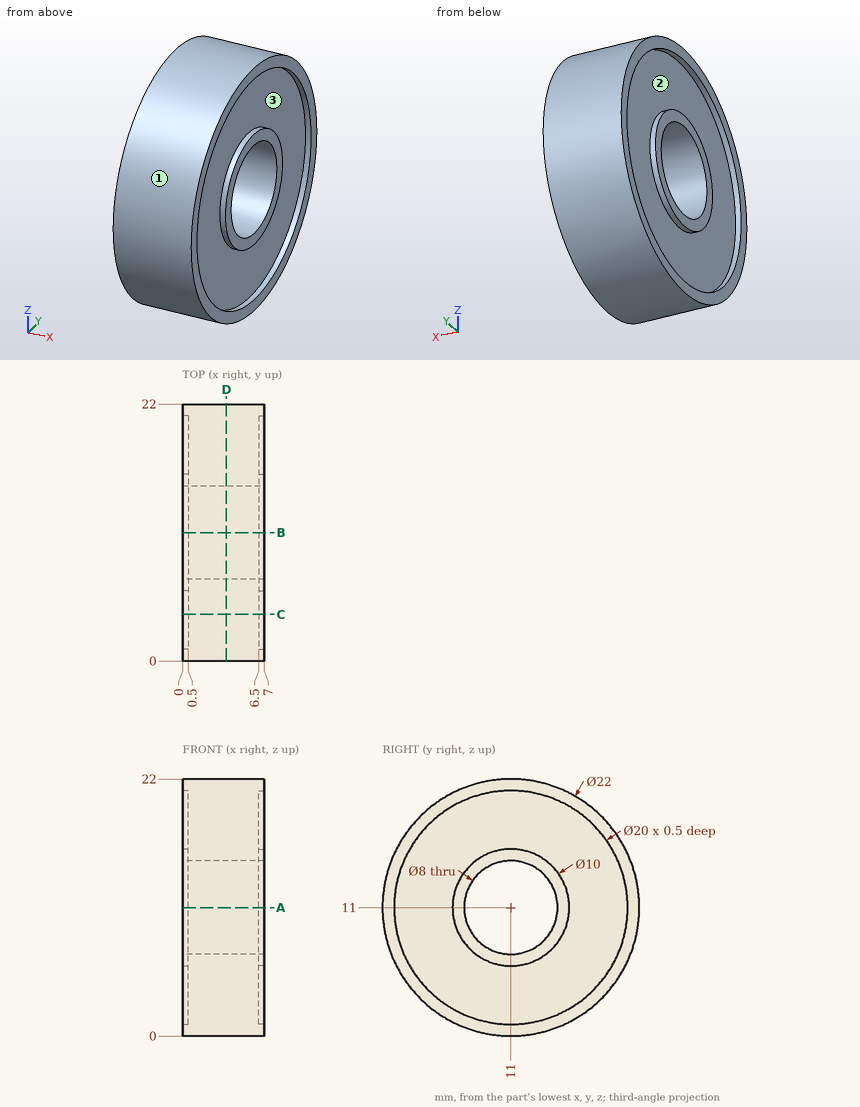
Answer from the drawing. Dimensions are ordinates in mm from the lowest x, y and z of the part. A direction names the side the tool comes from. Give positions to 0.01 mm unless a question says otherwise; leave off trailing zeros. Loops run counter-clockwise (first coordinate to the right, second up) from the corner with the lowest first, then second, coordinate; pieces in that order, holes last. Notation, with made-up numbers: (40.5, 30) -> (58.5, 30) arc R34 cw to (58.5, 62) -> close; hole circle Ø5 at (10.5, 29.25). An arc over 180 degrees is marked (long way). Answer as CSV lines item,"result".
Item 1: Find section C-C on y = 4. Give the vertices of the cut face in (x, z).
Returned:
outline,"(0, 2.51) -> (7, 2.51) -> (7, 3.86) -> (6.5, 3.86) -> (6.5, 18.14) -> (7, 18.14) -> (7, 19.49) -> (0, 19.49) -> (0, 18.14) -> (0.5, 18.14) -> (0.5, 3.86) -> (0, 3.86) -> close"
Item 2: Each of these flat-tipped pins is pushed along its axis until it touches: pin 1 (7 mm diameter, centred on y = 11, z = 11, fed in from +X); pin 2 (1.5 mm diameter, centred on x = 3, y = 10, fed in from +Z); pin 3 (2 mm diameter, centred on y = 18.5, z = 12, fed in from -X). Where does it stop, or does it pass through?
Returned:
pin 1,"passes through"
pin 2,"stops at z = 22"
pin 3,"stops at x = 0.5"
Item 3: Find section A-A on z = 11. Give the vertices of the cut face in (x, y), plus the area to 3 significant figures.
Returned:
outline,"(0, 0) -> (7, 0) -> (7, 1) -> (6.5, 1) -> (6.5, 6) -> (7, 6) -> (7, 7) -> (0, 7) -> (0, 6) -> (0.5, 6) -> (0.5, 1) -> (0, 1) -> close; (0, 15) -> (7, 15) -> (7, 16) -> (6.5, 16) -> (6.5, 21) -> (7, 21) -> (7, 22) -> (0, 22) -> (0, 21) -> (0.5, 21) -> (0.5, 16) -> (0, 16) -> close"
area,"88.0 mm²"
Item 4: Find section D-D on x = 3.75. Give the vertices of the cut face in (y, z), plus the area to 3 significant figures.
Returned:
outline,"circle Ø22 at (11, 11); hole circle Ø8 at (11, 11)"
area,"330 mm²"
Item 5: Consider line 1 (Z direction, x = 3.75, y = 11); line 2 (X direction, y = 16, z = 4.5); line 3 (Z direction, x = 1.5, y = 14). Determine where each line is inside the solid, lowest interval first. Write a range as [from, to].
Returned:
line 1,"z = [0, 7], [15, 22]"
line 2,"x = [0.5, 6.5]"
line 3,"z = [0.42, 8.35], [13.65, 21.58]"
Item 6: For the marked faces 1, 2 and 3, determine the directions among +Z, -Z, +X, -X, +Y, -Y from which every point of the face is accessible in a straight line to the end or side of a thin tool.
Returned:
face 1,"+X, -X"
face 2,"-X"
face 3,"+X"
